```python
from build123d import *

# Parameters (mm, degrees)
SKETCH1_W           = 127
SKETCH1_H           = 95.34985535
SKETCH1_R           = 3.2639
BOSS_EXTRUDE1_DEPTH = 9.525


with BuildPart() as part:
    # Sketch1 → Boss-Extrude1 (new body)
    with BuildSketch(Plane(origin=(0, 0, 0), x_dir=(1, 0, 0), z_dir=(0, 1, 0))):
        with Locations((1.506e-06, 55.24971147)):
            Rectangle(SKETCH1_W, SKETCH1_H)
        with Locations(Location((-50.8000007, 80.487207029, 0), (0, 0, 90))):
            Circle(SKETCH1_R, mode=Mode.SUBTRACT)
        with Locations(Location((50.800003712, 80.487207029, 0), (0, 0, 90))):
            Circle(SKETCH1_R, mode=Mode.SUBTRACT)
        with Locations(Location((50.800003712, 30.012215911, 0), (0, 0, 90))):
            Circle(SKETCH1_R, mode=Mode.SUBTRACT)
    extrude(amount=BOSS_EXTRUDE1_DEPTH)


solid = part.part
```
Can you work these out from the model? Positions are in its coordinate system, mm. Round coordinates to 2 decimals unless told otherwise and drop trailing zeros. Loops run counter-clockwise (first coordinate to the right, second up) from the corner with the lowest first, then second, coordinate; pieces in that order, holes last. Notation, with made-up numbers: M -7,80 L 0,80 A19 cw 0,85 Z; hole C 2,4 d6. An arc over 180 degrees is marked long. Answer as a JSON object with one key per item and string values. Group by question number.
Q1. We'd pull the mould along X, two halves only. Please class faces 1 (the cylindrical face through (53.696, 4.696, -31.518)), 2 (the flat face through (-1, 9.525, -56)), 3 (the flat face through (-63.5, 5, -55)), 4 (the cylindrical face through (52.05, 4.696, -83.502)): +X half, -X half, draft (parallel to the pull), parting line (faces both ways), or undercut.
Q2. Please list where these lines run through material, in increasing order: L1, parallel to Z at x = -50.8, y = 5; L2, parallel to Z at x = 52.5, y = 8.
Q3. Will this pin go through, and if not, where does the flat tip stop? pin 1 (4 mm diameter, centred on x = 50.8, z = -30.01, fed in from -Y).
Q4. Imagine slicing it at A-A, the plane x = -50.8. Please give me the cut outline in (y, z) (3 decimals), then the cut area to 3 significant figures.
Findings:
{
 "1": {"face 1": "undercut", "face 2": "draft", "face 3": "-X half", "face 4": "undercut"},
 "2": {"L1": "z = -102.92 to -83.75, -77.22 to -7.57", "L2": "z = -102.92 to -83.27, -77.7 to -32.8, -27.23 to -7.57"},
 "3": {"pin 1": "passes through"},
 "4": {"outline": "M 0,-102.925 L 9.525,-102.925 L 9.525,-83.751 L 0,-83.751 Z; M 0,-77.223 L 9.525,-77.223 L 9.525,-7.575 L 0,-7.575 Z", "area": "846 mm2"}
}
